Autodesk Inventor part; units mm, degrees
ref_plane "YZ Plane" through (0, 0, 0) normal (1, 0, 0) x (0, 1, 0)
ref_plane "XZ Plane" through (0, 0, 0) normal (0, 1, 0) x (-1, 0, 0)
ref_plane "XY Plane" through (0, 0, 0) normal (0, 0, 1) x (1, 0, 0)
sketch "Sketch1" plane through (0, 0, 0) normal (1, 0, 0) x (0, 1, 0)
  line L0 (59.5474, 107.5539) -> (-16.4526, 107.5539)
  line L1 (-16.4526, 107.5539) -> (-16.4526, 17.5539)
  line L2 (-16.4526, 17.5539) -> (59.5474, 17.5539)
  line L3 (59.5474, 17.5539) -> (59.5474, 107.5539)
  point P0 (0, 0)
  dimension "d0" = 90
  dimension "d1" = 76
extrude "Extrusion1" add sketch "Sketch1" along normal blind 3
sketch "Sketch2" plane through (3, 0, 0) normal (1, 0, 0) x (0, 0, -1)
  point P0 (0, 0)
sketch "Sketch3" plane through (3, 0, 0) normal (1, 0, 0) x (0, 0, -1)
  line L0 (-107.5539, -16.4526) -> (-17.5539, -16.4526)
  line L1 (-17.5539, -16.4526) -> (-17.5539, 59.5474)
  line L2 (-17.5539, 59.5474) -> (-107.5539, 59.5474)
  line L3 (-107.5539, 59.5474) -> (-107.5539, -16.4526)
  line L4 (-107.5539, 59.5474) -> (-17.5539, 59.5474)
  line L5 (-17.5539, 59.5474) -> (-17.5539, 53.5474)
  line L6 (-17.5539, 53.5474) -> (-107.5539, 53.5474)
  line L7 (-107.5539, 53.5474) -> (-107.5539, 59.5474)
  point P0 (0, 0)
  dimension "d4" = 6
extrude "Extrusion2" add sketch "Sketch3" along normal blind 4 contours L3 L2 L1 L6
sketch "Sketch5" plane through (0, 0, 0) normal (-1, 0, 0) x (0, 0, 1)
  line L0 (107.5539, -16.4526) -> (17.5539, -16.4526)
  line L1 (107.5539, 59.5474) -> (107.5539, -16.4526)
  line L2 (17.5539, 59.5474) -> (107.5539, 59.5474)
  line L3 (17.5539, -16.4526) -> (17.5539, 59.5474)
  line L4 (17.5539, -16.4526) -> (20.5539, -16.4526)
  line L5 (20.5539, -16.4526) -> (20.5539, -13.4526) construction
  line L6 (20.5539, -13.4526) -> (17.5539, -13.4526) construction
  line L7 (17.5539, -13.4526) -> (17.5539, -16.4526)
  circle A0 centre (20.5539, -13.4526) radius 1.5
  line L8 (107.5539, -16.4526) -> (104.5539, -16.4526)
  line L9 (104.5539, -16.4526) -> (104.5539, -13.4526)
  line L10 (104.5539, -13.4526) -> (107.5539, -13.4526)
  line L11 (107.5539, -13.4526) -> (107.5539, -16.4526)
  line L12 (17.5539, 59.5474) -> (20.5539, 59.5474)
  line L13 (20.5539, 59.5474) -> (20.5539, 56.5474)
  line L14 (20.5539, 56.5474) -> (17.5539, 56.5474)
  line L15 (17.5539, 56.5474) -> (17.5539, 59.5474)
  line L16 (107.5539, 59.5474) -> (104.5539, 59.5474)
  line L17 (104.5539, 59.5474) -> (104.5539, 56.5474)
  line L18 (104.5539, 56.5474) -> (107.5539, 56.5474)
  line L19 (107.5539, 56.5474) -> (107.5539, 59.5474)
  circle A1 centre (20.5539, 56.5474) radius 1.8641
  circle A2 centre (104.5539, 56.5474) radius 1.8641
  circle A3 centre (104.5539, -13.4526) radius 1.5
  point P0 (0, 0)
  dimension "d7" = 3
  dimension "d9" = 3
extrude "Extrusion3" cut sketch "Sketch5" against normal up to surface (7 mm away) contours A3 L10 L9 | L9 L10 A3 | A2 L17 L18 | L18 L17 A2 | A1 L13 L14 | L14 L13 A1 | A0
CAD build for the part. Positions are in the model's coordinates, mm. Round coordinates to 2 decimals unless told otherwise and drop trailing zeros. Order: outer loops, then holes, each group sorted by start corner. A loop starts at its lowest first (then second) coordinate and runs counter-clockwise, first axis right, second up. Notation, with made-up numbers: M 33,-18 L 55,-18 A13 cw 55,-13 Z; hole C 74.25,1 d2. An arc over 180 degrees is marked long. Use one line per item in the form item = value.
Q1. Saw through at A-A on z = 50. Give the cut face in (x, y).
Recorded:
outline = M 0,-16.45 L 3,-16.45 L 3,53.55 L 7,53.55 L 7,59.55 L 0,59.55 Z
Q2. Probe L1, parallel to Y at x = 3.5, z = 29; L2, parallel to X at y = -3, z = 28; L3, parallel to Z at x = 3.25, y = 55.5. List the from-to ranges inside material, lowest first.
Recorded:
L1 = 53.55 to 59.55
L2 = 0 to 3
L3 = 17.55 to 19.01, 22.1 to 103.01, 106.1 to 107.55
Q3. Two-plate mould, pull along Y, no slides. Class faces 1 (the cylindrical face through (1.479, -13.387, 103.055)), 2 (the flat face through (3, 59.547, 62)), 3 (the flat face through (5, 53.547, 62)), 4 (the flat face through (3, 18, 63)): +Y half, -Y half, draft (parallel to the pull), parting line (faces both ways), or undercut.
Recorded:
face_1 = undercut
face_2 = +Y half
face_3 = -Y half
face_4 = draft
Q4. Saw through at C-C on y = 34.5. Give the cut face in (x, z), then the cut area to 3 significant figures.
Recorded:
outline = M 0,17.55 L 3,17.55 L 3,107.55 L 0,107.55 Z
area = 270 mm^2
Q5. Flat gauge pins, fed straight in: P1, Ø21, axis at y = 22.5, z = 76, coming from the +X side; P2, Ø3, axis at x = 5.5, z = 82, coming from the -Y side. Where does each tip first touch, or does it go through?
Recorded:
P1 = 3
P2 = 53.55
Q6. Saw through at B-B on x = 4.25. Give the cut face in (y, z).
Recorded:
outline = M 53.55,17.55 L 59.55,17.55 L 59.55,107.55 L 53.55,107.55 Z; hole C 56.55,20.55 d3.73; hole C 56.55,104.55 d3.73
